```python
from build123d import *

# Parameters (mm, degrees)
SKETCH1_R            = 1
BOSS_EXTRUDE1_DEPTH  = 6
SKETCH2_R            = 2.6
CUT_EXTRUDE1_DEPTH   = 6
SKETCH3_W            = 7.6
SKETCH3_H            = 13
BOSS_EXTRUDE2_DEPTH  = 6
BOSS_EXTRUDE5_START  = -5
SKETCH6_W            = 3
SKETCH6_H            = 2
BOSS_EXTRUDE5_DEPTH  = 13
BOSS_EXTRUDE6_START  = -7.5
SKETCH10_R           = 4
SKETCH10_R_2         = 2.6
BOSS_EXTRUDE6_DEPTH  = 1.5
BOSS_EXTRUDE7_START  = -6
SKETCH12_R           = 2.6
SKETCH12_R_2         = 2.4
BOSS_EXTRUDE7_DEPTH  = 2
CUT_EXTRUDE2_DEPTH   = 7
SKETCH14_W           = 3
SKETCH14_H           = 6
CUT_EXTRUDE3_DEPTH   = 2
SKETCH15_W           = 0.2
SKETCH15_H           = 13
CUT_EXTRUDE5_DEPTH   = 7.5
SKETCH16_W           = 3
SKETCH16_H           = 3
CUT_EXTRUDE6_DEPTH   = 3
SKETCH17_W           = 2.8
SKETCH17_H           = 2.8
BOSS_EXTRUDE9_DEPTH  = 3
BOSS_EXTRUDE10_START = 24.4
SKETCH17_2_W         = 2.8
SKETCH17_2_H         = 2.8
BOSS_EXTRUDE10_DEPTH = 3
SKETCH18_W           = 37.3
SKETCH18_H           = 13
CUT_EXTRUDE11_DEPTH  = 9
SKETCH20_W           = 2.8
SKETCH20_H           = 2.8
BOSS_EXTRUDE11_DEPTH = 3


with BuildPart() as part:
    # Sketch1 → Boss-Extrude1 (new body)
    with BuildSketch(Plane.XY):
        with BuildLine():
            ThreePointArc((3.75, -5), (4.47902769, -4.358991965), (5.1, -3.61282438))
            Line((5.1, -3.61282438), (5.1, 3.61282438))
            ThreePointArc((5.1, 3.61282438), (0, 6.25), (-5.1, 3.61282438))
            Line((-5.1, 3.61282438), (-5.1, -3.61282438))
            ThreePointArc((-5.1, -3.61282438), (-4.47902769, -4.358991965), (-3.75, -5))
            Line((-3.75, -5), (-14.7, -5))
            Line((-14.7, -5), (-14.7, 8))
            Line((-14.7, 8), (14.7, 8))
            Line((14.7, 8), (14.7, -5))
            Line((14.7, -5), (3.75, -5))
        make_face()
        with Locations((11.5, 0)):
            Circle(SKETCH1_R, mode=Mode.SUBTRACT)
        with Locations((-11.5, 0)):
            Circle(SKETCH1_R, mode=Mode.SUBTRACT)
    extrude(amount=BOSS_EXTRUDE1_DEPTH)

    # Sketch2 → Cut-Extrude1 (cut)
    with BuildSketch(Plane.XY):
        with Locations((-11.5, 0)):
            Circle(SKETCH2_R)
        with Locations((11.5, 0)):
            Circle(SKETCH2_R)
    extrude(amount=CUT_EXTRUDE1_DEPTH, mode=Mode.SUBTRACT)

    # Sketch3 → Boss-Extrude2 (add)
    with BuildSketch(Plane.XY):
        with Locations((-18.5, 1.5)):
            Rectangle(SKETCH3_W, SKETCH3_H)
    extrude(amount=BOSS_EXTRUDE2_DEPTH)

    # Sketch6 → Boss-Extrude5 (add)
    with BuildSketch(Plane(origin=(0, 0, 0), x_dir=(1, 0, 0), z_dir=(0, 1, 0)).offset(BOSS_EXTRUDE5_START)):
        with Locations((-23.8, -3)):
            Rectangle(SKETCH6_W, SKETCH6_H)
        with Locations((16.2, -3)):
            Rectangle(SKETCH6_W, SKETCH6_H)
    extrude(amount=BOSS_EXTRUDE5_DEPTH)

    # Sketch10 → Boss-Extrude6 (add)
    with BuildSketch(Plane.XY.offset(6).offset(BOSS_EXTRUDE6_START)):
        with Locations((-11.5, 0)):
            Circle(SKETCH10_R)
        with Locations((-11.5, 0)):
            Circle(SKETCH10_R_2, mode=Mode.SUBTRACT)
        with BuildLine():
            Line((14.7, 2.4), (14.7, -2.4))
            ThreePointArc((14.7, -2.4), (7.5, 0), (14.7, 2.4))
        make_face()
        with Locations((11.5, 0)):
            Circle(SKETCH10_R_2, mode=Mode.SUBTRACT)
    extrude(amount=BOSS_EXTRUDE6_DEPTH)

    # Sketch12 → Boss-Extrude7 (add)
    with BuildSketch(Plane(origin=(0, 0, 0), x_dir=(-1, 0, 0), z_dir=(0, 0, -1)).offset(BOSS_EXTRUDE7_START)):
        with Locations((11.5, 0)):
            Circle(SKETCH12_R)
        with Locations((11.5, 0)):
            Circle(SKETCH12_R_2, mode=Mode.SUBTRACT)
        with Locations((-11.5, 0)):
            Circle(SKETCH12_R)
        with Locations((-11.5, 0)):
            Circle(SKETCH12_R_2, mode=Mode.SUBTRACT)
    extrude(amount=BOSS_EXTRUDE7_DEPTH)

    # Sketch13 → Cut-Extrude2 (cut)
    with BuildSketch(Plane.XZ.offset(5)):
        Polygon((-22.3, 0), (-16.3, 0), (-16.3, 2), (-17.8, 2), (-17.8, 6), (-20.8, 6), (-20.8, 2), (-22.3, 2), align=None)
    extrude(amount=-CUT_EXTRUDE2_DEPTH, mode=Mode.SUBTRACT)

    # Sketch14 → Cut-Extrude3 (cut)
    with BuildSketch(Plane(origin=(0, 0, 0), x_dir=(-1, 0, 0), z_dir=(0, 0, -1))):
        with Locations((19.3, 5)):
            Rectangle(SKETCH14_W, SKETCH14_H)
    extrude(amount=-CUT_EXTRUDE3_DEPTH, mode=Mode.SUBTRACT)

    # Sketch15 → Cut-Extrude5 (cut, symmetric)
    with BuildSketch(Plane.XY):
        with Locations((-12.1, 1.5)):
            Rectangle(SKETCH15_W, SKETCH15_H)
        with Locations((12.1, 1.5)):
            Rectangle(SKETCH15_W, SKETCH15_H)
    extrude(amount=CUT_EXTRUDE5_DEPTH, both=True, mode=Mode.SUBTRACT)

    # Sketch16 → Cut-Extrude6 (cut)
    with BuildSketch(Plane(origin=(12, 0, 0), x_dir=(0, 0, -1), z_dir=(1, 0, 0))):
        with Locations((-3, 5.173669459)):
            Rectangle(SKETCH16_W, SKETCH16_H)
    cut_extrude6 = extrude(amount=-CUT_EXTRUDE6_DEPTH, mode=Mode.SUBTRACT)

    # Mirror1: Cut-Extrude6 across plane
    add(cut_extrude6.mirror(Plane(origin=(0, 0, 0), x_dir=(0, 0, 1), z_dir=(1, 0, 0))), mode=Mode.SUBTRACT)

    # Sketch17 → Boss-Extrude9 (add)
    with BuildSketch(Plane(origin=(-12.2, 0, 0), x_dir=(0, 0, -1), z_dir=(1, 0, 0))):
        with Locations((-3, 5.173669459)):
            Rectangle(SKETCH17_W, SKETCH17_H)
    extrude(amount=BOSS_EXTRUDE9_DEPTH)

    # Sketch17<2> → Boss-Extrude10 (add)
    with BuildSketch(Plane(origin=(-12.2, 0, 0), x_dir=(0, 0, -1), z_dir=(1, 0, 0)).offset(BOSS_EXTRUDE10_START)):
        with Locations((-3, 5.173669459)):
            Rectangle(SKETCH17_2_W, SKETCH17_2_H)
    extrude(amount=-BOSS_EXTRUDE10_DEPTH)

    # Sketch18 → Cut-Extrude11 (cut, symmetric)
    with BuildSketch(Plane.XY):
        with Locations((-6.65, 1.5)):
            Rectangle(SKETCH18_W, SKETCH18_H)
    extrude(amount=CUT_EXTRUDE11_DEPTH, both=True, mode=Mode.SUBTRACT)

    # Sketch20 → Boss-Extrude11 (add)
    with BuildSketch(Plane.ZY.offset(-12.2)):
        with Locations((3, 5.173669459)):
            Rectangle(SKETCH20_W, SKETCH20_H)
    extrude(amount=BOSS_EXTRUDE11_DEPTH)


solid = part.part
```
Geometry check sheet. Reference: the model listing, model coordinates, mm. A direction names the side the tool comes from. Coordinates: 2 decimals unless noted, no trailing zeros. Write each loop counter-clockwise with the first axis right and the second up, starting at its lowest first coordinate (ties: lowest second). Pieces come first, ordered by that corner, then holes. Notation, with made-up numbers: M 87.25,68 L 117.25,68 A19 cw 117.25,80 Z; hole C -16,-3 d11. An arc over 180 degrees is marked long. Answer as a JSON object with one key per item and string values.
1. Section check B-B, the plane z = 3.75. Enter the section's corners in (x, y).
Answers below:
{"outline": "M 9.2,3.77 L 12.2,3.77 L 12.2,2.5 A2.6 cw 12.2,-2.5 L 12.2,-5 L 17.7,-5 L 17.7,8 L 12.2,8 L 12.2,6.57 L 9.2,6.57 Z"}
2. Draft check along Y on faces 6 (the flat face through (14.7, 2, 1)), 7 (the cylindrical face through (14.1, 0, 1.2)), 8 (the cylindrical face through (13.578, 3.418, -0.76)). Enter one of: released by +Y, released by -Y, zero draft, split by the parting line, or undercut.
Answers below:
{"face 6": "zero draft", "face 7": "undercut", "face 8": "released by +Y"}
3. Section check A-A, the plane y = 0. Enter the section's corners in (x, z), plus the area to 3 significant figures.
Answers below:
{"outline": "M 13.9,4 L 14.1,4 L 14.1,-1.5 L 14.7,-1.5 L 14.7,2 L 17.7,2 L 17.7,4 L 14.7,4 L 14.7,6 L 13.9,6 Z", "area": "10.9 mm²"}
4. Section check C-C, the plane x = 13.25. Enter the section's corners in (y, z), plus the area to 3 significant figures.
Answers below:
{"outline": "M -5,0 L -3.6,0 L -3.6,-1.5 L -1.92,-1.5 L -1.92,4 L -1.64,4 L -1.64,6 L -5,6 Z; M 1.64,4 L 1.92,4 L 1.92,-1.5 L 3.6,-1.5 L 3.6,0 L 8,0 L 8,6 L 1.64,6 Z", "area": "61.1 mm²"}
5. Go/stop test with flat-tipped pins: pin 1 Ø1.8 at (y, z) = (1.5, 0.5) entering from +X; pin 2 Ø0.8 at (x, y) = (11, 5) entering from +Z; pin 3 Ø2 at (x, y) = (13.5, 5.5) entering from -Z. Record where each tip stops, or that it passes through.
Answers below:
{"pin 1": "stops at x = 14.7", "pin 2": "stops at z = 4.4", "pin 3": "stops at z = 0"}
6. Tool access check on faces 1 (the flat face through (14.7, 2, 5)), 2 (the flat face through (14, -4, 0)), 3 (the flat face through (11, 5, 1.6)), 4 (the flat face through (12.2, -4, 3)), 5 (the flat face through (16, 1, 2)). Record the directions out of +Z, -Z, +X, -X, +Y, -Y that give a thin tool (end or side, any length) a straight path to the whole face; none if there is none.
Answers below:
{"face 1": "+Z, +X, +Y, -Y", "face 2": "-Z, +X, -Y", "face 3": "-Z, -X, +Y, -Y", "face 4": "+Z, -Z, -X, -Y", "face 5": "-Z, +X, +Y, -Y"}
7. Scan lines: L1, parallel to Y at x = 12, z = 3.5; L2, parallel to Z at x = 15.5, y = 7; L3, parallel to Z at x = 13.5, y = -3.75. Record each from-to range of solid material in increasing order.
Answers below:
{"L1": "y = 3.77 to 6.57", "L2": "z = 2 to 4", "L3": "z = 0 to 6"}
8. Section check D-D, the plane y = 5.75. Enter the section's corners in (x, z).
Answers below:
{"outline": "M 9.2,1.6 L 12.2,1.6 L 12.2,0 L 14.7,0 L 14.7,2 L 17.7,2 L 17.7,4 L 14.7,4 L 14.7,6 L 12.2,6 L 12.2,4.4 L 9.2,4.4 Z"}
